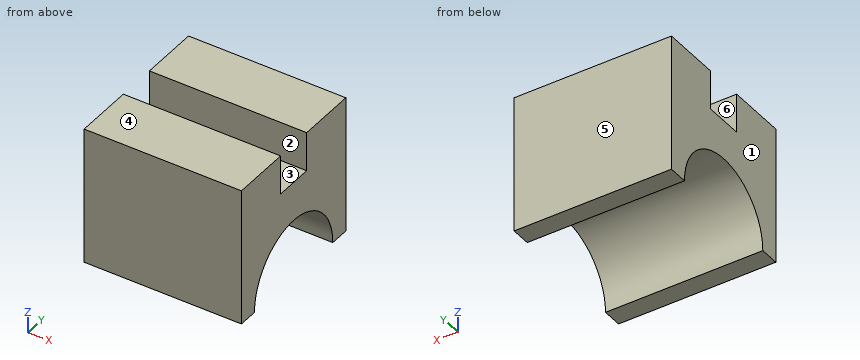
```python
from build123d import *

# Parameters (mm, degrees)
F0_W     = 40
F0_H     = 35
F1_DEPTH = 20
F3_DEPTH = 100
F2_W     = 10
F2_H     = 10
F4_DEPTH = 40.001


with BuildPart() as f1:
    # F0 (on Front) → F1 (new body, symmetric)
    with BuildSketch(Plane.XZ):
        with Locations((0, 17.5)):
            Rectangle(F0_W, F0_H)
    extrude(amount=F1_DEPTH, both=True)

    # F2 (on face) → F3 (cut, symmetric)
    with BuildSketch(Plane(origin=(-20, 0, 0), x_dir=(0, -1, 0), z_dir=(-1, 0, 0))):
        with BuildLine():
            Line((-15, 0), (15, 0))
            ThreePointArc((15, 0), (0, 15), (-15, 0))
        make_face()
    extrude(amount=F3_DEPTH, both=True, mode=Mode.SUBTRACT)

    # F2 (on face) → F4 (cut, through all)
    with BuildSketch(Plane(origin=(-20, 0, 0), x_dir=(0, -1, 0), z_dir=(-1, 0, 0))):
        with Locations((0, 30)):
            Rectangle(F2_W, F2_H)
    extrude(amount=-F4_DEPTH, mode=Mode.SUBTRACT)


solid = f1.part
```
Here's how the part is built. I have some questions about the finished solid (model axes, mm). Face numbers are marked on the shaded views. A direction names the side the tool comes from. Round coordinates to 2 decimals unless told otherwise and drop trailing zeros. Order: outer loops, then holes, each group sorted by start corner. A loop starts at its lowest first (then second) coordinate and runs counter-clockwise, first axis right, second up. Notation, with made-up numbers: (-20.75, -10) -> (26.25, -10) arc R13 ccw to (26.25, -6) -> close; hole circle Ø11 at (-23, 62.5). An arc over 180 degrees is marked (long way). Use a Markdown table: item, result. Add a question column.
(1) If we mould it in two halves opening along Y, with no side actions, what happens to the marked faces 3, 4, 5 and 6? For each: released by +Y, released by -Y, zero draft, split by the parting line, or undercut.
(2) I need wall thicknesses on line 1 along Y through (x, z) = (7, 33); line 2 along Y through (x, z) = (3, 12); line 3 along Z through (x, y) = (-5.5, 9.5). Which ranges of each line are inside material? Lowest first, please.
(3) For pin 1 Ø5 at (x, y) = (4.5, 0.5) entering from +Z; pin 2 Ø1.5 at (x, y) = (-12, -13) entering from -Z; pin 3 Ø1.5 at (x, y) = (-15.5, 1.5) entering from -Z, each with a flat end and sliding along its axis, tell me the tip position at first contact or that it passes through.
(4) Suppose I cut it at B-B, the plane y = 0. Please give me the cut outline in (x, z).
(5) Suppose I cut it at A-A, the plane x = -9. Please give me the cut outline in (y, z), and give its area (3 significant figures).
(6) For the marked faces 1 and 2, which set-ups out of +Z, -Z, +X, -X, +Y, -Y let a thin tool reach every point of the face, with its end or its side?
(7) Suppose I cut it at C-C, the plane y = -6. Please give me the cut outline in (x, z), and give its area (3 significant figures).
Verdict:
| question | item | result |
|---|---|---|
| 1 | face 3 | undercut |
| 1 | face 4 | zero draft |
| 1 | face 5 | released by +Y |
| 1 | face 6 | undercut |
| 2 | line 1 | -20 to -5, 5 to 20 |
| 2 | line 2 | -20 to -9, 9 to 20 |
| 2 | line 3 | 11.61 to 35 |
| 3 | pin 1 | z = 25 |
| 3 | pin 2 | z = 5.99 |
| 3 | pin 3 | z = 14.83 |
| 4 | outline | (-20, 15) -> (20, 15) -> (20, 25) -> (-20, 25) -> close |
| 5 | outline | (-20, 0) -> (-15, 0) arc R15 cw to (15, 0) -> (20, 0) -> (20, 35) -> (5, 35) -> (5, 25) -> (-5, 25) -> (-5, 35) -> (-20, 35) -> close |
| 5 | area | 947 mm2 |
| 6 | face 1 | +Z, -Z, -X, +Y, -Y |
| 6 | face 2 | +Z, +X, -X |
| 7 | outline | (-20, 13.75) -> (20, 13.75) -> (20, 35) -> (-20, 35) -> close |
| 7 | area | 850 mm2 |
